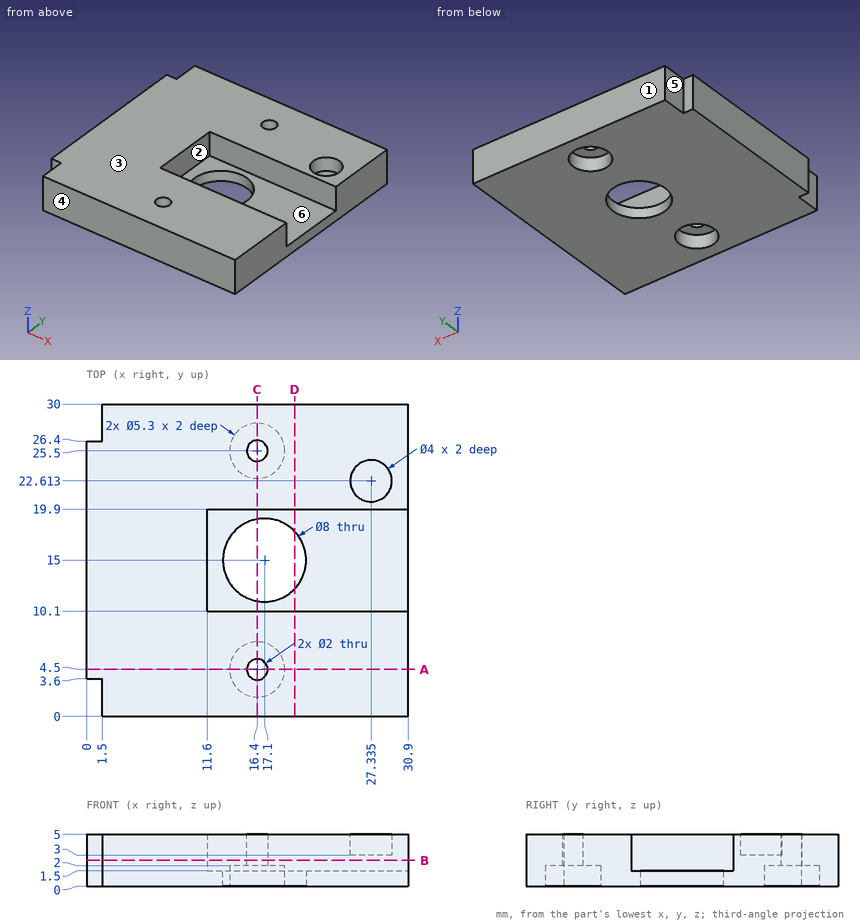
Here's the drawing with two shaded views (mm, measured from the low corner). I have some questions. A direction names the side the tool comes from. Give positions to 0.01 mm unless a question says otherwise; leave off trailing zeros. Order: outer loops, then holes, each group sorted by start corner. A loop starts at its lowest first (then second) coordinate and runs counter-clockwise, first axis right, second up. Notation, with made-up numbers: (43, 20) -> (65, 20) arc R7 ccw to (65, 27) -> close; hole circle Ø5 at (-29.5, 81). An arc over 180 degrees is marked (long way). One line per item, written item: value. Start each with the question number.
1. I need wall thicknesses on probe 1 along Y at (x, z) = (13, 2.65); probe 2 along Y at (x, z) = (16.4, 0.7); probe 3 along Y at (x, z) = (16.4, 3). Which ranges of each line are inside material? Lowest first, please. Write a range as from..to.
2. For the marked faces 4, 5 and 6, which set-ups out of +Z, -Z, +X, -X, +Y, -Y let a thin tool reach every point of the face, with its end or its side?
3. Imagine slicing it at D-D, the plane x = 20. List the corners of the cut face in (y, z) for me (3 decimals).
4. Imagine slicing it at A-A, the plane y = 4.5. List the corners of the cut face in (x, z) for me.
5. Imagine slicing it at B-B, the plane z = 2.5. List the corners of the cut face in (x, y) for me, plus the area to 3 significant figures.
6. Will these pins go through, and if not, where does the flat tip stop? pin 1 Ø0.8 at (x, z) = (1, 3.5) entering from -Y; pin 2 Ø5 at (x, y) = (17.1, 15) entering from -Z; pin 3 Ø2 at (x, y) = (17.5, 5) entering from -Z; pin 4 Ø4 at (x, y) = (20, 14.5) entering from +Z.
7. Imagine slicing it at C-C, the plane x = 16.4. List the corners of the cut face in (y, z) for me.
8. We'd pull the mould along Y, two halves only. Please class the marked faces 1, 2 and 3: released by +Y, released by -Y, zero draft, split by the parting line, or undercut.
Values follow:
1. probe 1: y = 0..10.1, 19.9..30
1. probe 2: y = 0..1.85, 7.15..11.06, 18.94..22.85, 28.15..30
1. probe 3: y = 0..3.5, 5.5..10.1, 19.9..24.5, 26.5..30
2. face 4: +Z, -Z, +X, -X, -Y
2. face 5: +Z, -Z, -X, +Y
2. face 6: +Z, +X
3. outline: (0, 0) -> (12.245, 0) -> (12.245, 1.5) -> (10.1, 1.5) -> (10.1, 5) -> (0, 5) -> close; (17.755, 0) -> (30, 0) -> (30, 5) -> (19.9, 5) -> (19.9, 1.5) -> (17.755, 1.5) -> close
4. outline: (0, 0) -> (13.75, 0) -> (13.75, 2) -> (15.4, 2) -> (15.4, 5) -> (0, 5) -> close; (17.4, 2) -> (19.05, 2) -> (19.05, 0) -> (30.9, 0) -> (30.9, 5) -> (17.4, 5) -> close
5. outline: (0, 3.6) -> (1.5, 3.6) -> (1.5, 0) -> (30.9, 0) -> (30.9, 10.1) -> (11.6, 10.1) -> (11.6, 19.9) -> (30.9, 19.9) -> (30.9, 30) -> (1.5, 30) -> (1.5, 26.4) -> (0, 26.4) -> close; hole circle Ø2 at (16.4, 4.5); hole circle Ø2 at (16.4, 25.5)
5. area: 721 mm2
6. pin 1: stops at y = 3.6
6. pin 2: passes through
6. pin 3: stops at z = 2
6. pin 4: stops at z = 1.5
7. outline: (0, 0) -> (1.85, 0) -> (1.85, 2) -> (3.5, 2) -> (3.5, 5) -> (0, 5) -> close; (5.5, 2) -> (7.15, 2) -> (7.15, 0) -> (11.06, 0) -> (11.06, 1.5) -> (10.1, 1.5) -> (10.1, 5) -> (5.5, 5) -> close; (18.94, 0) -> (22.85, 0) -> (22.85, 2) -> (24.5, 2) -> (24.5, 5) -> (19.9, 5) -> (19.9, 1.5) -> (18.94, 1.5) -> close; (26.5, 2) -> (28.15, 2) -> (28.15, 0) -> (30, 0) -> (30, 5) -> (26.5, 5) -> close
8. face 1: released by +Y
8. face 2: undercut
8. face 3: zero draft
